from build123d import *

# Parameters (mm, degrees)
F1_DEPTH  = 38
F3_DEPTH  = 25
F4_DEPTH  = 38
F0_W      = 5
F0_H      = 28
F5_DEPTH  = 38
F6_DEPTH  = 34
F7_DEPTH  = 14
F0_W_2    = 8.5
F0_H_2    = 23
F8_DEPTH  = 29
F9_DEPTH  = 24
F0_W_3    = 25
F10_DEPTH = 19
F11_DEPTH = 10
F0_H_3    = 10
F12_DEPTH = 5


with BuildPart() as f1:
    # F0 (on Top) → F1 (new body)
    with BuildSketch(Plane.XY):
        Polygon((-33.5, -24), (-33.5, -14), (-33.5, -4), (-33.5, 19), (-38.5, 19), (-38.5, -24), align=None)
    extrude(amount=F1_DEPTH)

    # F2 (on face) → F3 (cut)
    with BuildSketch(Plane.YZ.offset(-33.5)):
        Polygon((-24, 38), (-24, 14), (19, 38), align=None)
    extrude(amount=-F3_DEPTH, mode=Mode.SUBTRACT)

    # F0 (on Top) → F4 (join)
    with BuildSketch(Plane.XY):
        Polygon((8.5, 19), (8.5, 24), (-38.5, 24), (-38.5, 19), (-33.5, 19), (-8.5, 19), (0, 19), align=None)
    extrude(amount=F4_DEPTH)



with BuildPart() as f5:
    # F0 (on Top) → F5 (new body)
    with BuildSketch(Plane.XY):
        with Locations((36, 10)):
            Rectangle(F0_W, F0_H)
    extrude(amount=F5_DEPTH)


with BuildPart() as f1_1:
    add(f1.part)

    add(f5.part)  # F6 merges F5
    # F0 (on Top) → F6 (join)
    with BuildSketch(Plane.XY):
        Polygon((8.5, -4), (33.5, -4), (33.5, 24), (8.5, 24), (8.5, 19), align=None)
    extrude(amount=F6_DEPTH)

    # F0 (on Top) → F7 (join)
    with BuildSketch(Plane.XY):
        Polygon((33.5, -24), (38.5, -24), (38.5, -4), (33.5, -4), (33.5, -14), align=None)
    extrude(amount=F7_DEPTH)

    # F0 (on Top) → F8 (join)
    with BuildSketch(Plane.XY):
        with Locations((4.25, 7.5)):
            Rectangle(F0_W_2, F0_H_2)
    extrude(amount=F8_DEPTH)

    # F0 (on Top) → F9 (join)
    with BuildSketch(Plane.XY):
        with Locations((-4.25, 7.5)):
            Rectangle(F0_W_2, F0_H_2)
    extrude(amount=F9_DEPTH)

    # F0 (on Top) → F10 (join)
    with BuildSketch(Plane.XY):
        with Locations((-21, 7.5)):
            Rectangle(F0_W_3, F0_H_2)
    extrude(amount=F10_DEPTH)

    # F0 (on Top) → F11 (join)
    with BuildSketch(Plane.XY):
        Polygon((-8.5, -14), (33.5, -14), (33.5, -4), (8.5, -4), (0, -4), (-8.5, -4), (-33.5, -4), (-33.5, -14), align=None)
    extrude(amount=F11_DEPTH)

    # F0 (on Top) → F12 (join)
    with BuildSketch(Plane.XY):
        with Locations((-21, -19)):
            Rectangle(F0_W_3, F0_H_3)
    extrude(amount=F12_DEPTH)


solid = f1_1.part
For this review, take the finished solid that the model builds, in its own axes (mm). A direction names the side the tool comes from. Round coordinates to 2 decimals unless told otherwise and drop trailing zeros. Loops run counter-clockwise (first coordinate to the right, second up) from the corner with the lowest first, then second, coordinate; pieces in that order, holes last. Notation, with made-up numbers: (8, 25) - (63, 25) arc R21 ccw to (63, 42) - close; hole circle Ø5 at (55.5, -28.75). An arc over 180 degrees is marked (long way). Put each result on its own line as item: value. Start each with the question number.
1. Consider section A-A on x = -24. State the section outline as (y, z) points.
2. Mouldability with a two-part tool opening along X and no side actions: class faces 4 (the flat face through (10, -4, 21)), 5 (the flat face through (-33.5, -3, 21)), 6 (the flat face through (36, -14, 14)) as +X half, -X half, draft (parallel to the pull), parting line (faces both ways), or undercut.
3. Consider section D-D on y = 17. State the section outline as (x, z) points.
4. Consider section B-B on z = 11. State the section outline as (x, y) points, plus the area to 3 significant figures.
5. For probe 1 along X at (y, z) = (12, 28); probe 2 along X at (y, z) = (19.5, 35.5); probe 3 along Z at (x, y) = (-21.5, 12), list the stretches that pass through material, from the lowest coordinate up. Write a range as [from, to].
6. For faces 1 (the flat face through (33.5, 10, 36)), 2 (the flat face through (4, 8, 29)), 3 (the flat face through (-8.5, -19, 2)), list the 3-axis set-ups (+Z, -Z, +X, -X, +Y, -Y) from which the entire face can be reached by the end or side of a thin tool; tool diameter is ignored.
7. Consider section C-C on z = 35. State the section outline as (x, y) points (3 decimals).
8. Insertion check: P1, Ø7, axis at x = 2, y = 6, coming from the +Z side; P2, Ø12.5, axis at x = 19.5, y = 4.5, coming from the +Z side; P3, Ø4.5, axis at y = 7.5, z = 36, coming from the -X side. Each pin has a flat end and moves straight along its axis. Give the tip position at first contact, or say it passes through.
Result sheet:
1. outline: (-24, 0) - (24, 0) - (24, 38) - (19, 38) - (19, 19) - (-4, 19) - (-4, 10) - (-14, 10) - (-14, 5) - (-24, 5) - close
2. face 4: undercut
2. face 5: undercut
2. face 6: draft
3. outline: (-38.5, 0) - (38.5, 0) - (38.5, 38) - (33.5, 38) - (33.5, 34) - (8.5, 34) - (8.5, 29) - (0, 29) - (0, 24) - (-8.5, 24) - (-8.5, 19) - (-33.5, 19) - (-33.5, 36.88) - (-38.5, 36.88) - close
4. outline: (-38.5, -24) - (-33.5, -24) - (-33.5, -4) - (33.5, -4) - (33.5, -24) - (38.5, -24) - (38.5, 24) - (-38.5, 24) - close
4. area: 2,360 mm^2
5. probe 1: [-38.5, -33.5], [0, 38.5]
5. probe 2: [-38.5, 8.5], [33.5, 38.5]
5. probe 3: [0, 19]
6. face 1: +Z, +Y, -Y
6. face 2: +Z, -Y
6. face 3: +Z, -Z, -Y
7. outline: (-38.5, 13.625) - (-33.5, 13.625) - (-33.5, 19) - (8.5, 19) - (8.5, 24) - (-38.5, 24) - close; (33.5, -4) - (38.5, -4) - (38.5, 24) - (33.5, 24) - close
8. P1: z = 29
8. P2: z = 34
8. P3: x = 8.5
